Geometry check sheet. Reference: the model listing, model coordinates, mm. Face numbers are marked on the shaded views. A direction names the side the tool comes from. Give positions to 0.01 mm unless a question says otherwise; leave off trailing zeros. Write each loop counter-clockwise with the first axis right and the second up, starting at its lowest first coordinate (ties: lowest second). Pieces come first, ordered by that corner, then holes. Notation, with made-up numbers: M 24.25,60.5 L 83.25,60.5 A22 ccw 83.25,84.5 Z; hole C -16.5,75.5 d2. An arc over 180 degrees is marked long. Write each question's results on one line, items separated by ' | '.
```python
from build123d import *

# Parameters (mm, degrees)
SKETCH_1_R               = 15
SKETCH_1_R_2             = 9
EXTRUDE_1_DEPTH          = 30
SKETCH_2_R               = 100
SKETCH_2_R_2             = 15
SKETCH_2_R_3             = 9
EXTRUDE_2_DEPTH          = 7
CUT_EXTRUDE_1_DEPTH      = 147.181394165
PATTERN_CIRCULAR_1_COUNT = 6
FILLET_1_R               = 10
HOLE_WIZARD_M30_1_D      = 26.5
HOLE_WIZARD_M30_1_DEPTH  = 62.538596798
HOLE_WIZARD_M30_1_TIP    = 7.961403202
CHAMFER_1_SIZE           = 5
CUT_EXTRUDE_1_2_DEPTH    = 145.568322948
PATTERN_CIRCULAR_2_COUNT = 4
FILLET_2_R               = 3


with BuildPart() as part:
    # 草图1 → 凸台-拉伸1 (new body)
    with BuildSketch(Plane(origin=(0, 0, 0), x_dir=(1, 0, 0), z_dir=(0, 1, 0))):
        with Locations(Location((0, 0, 0), (0, 0, 270))):
            Circle(SKETCH_1_R)
        with Locations(Location((0, 0, 0), (0, 0, 270))):
            Circle(SKETCH_1_R_2, mode=Mode.SUBTRACT)
    extrude(amount=EXTRUDE_1_DEPTH)

    # 草图2 → 凸台-拉伸2 (add)
    # profile 1 of 2: a face of its own
    with BuildSketch(Plane(origin=(0, 30, 0), x_dir=(1, 0, 0), z_dir=(0, 1, 0))):
        with Locations(Location((0, 0, 0), (0, 0, 270))):
            Circle(SKETCH_2_R)
        with Locations(Location((0, 0, 0), (0, 0, 270))):
            Circle(SKETCH_2_R_2, mode=Mode.SUBTRACT)
    # profile 2 of 2: a face of its own
    with BuildSketch(Plane(origin=(0, 30, 0), x_dir=(1, 0, 0), z_dir=(0, 1, 0))):
        with Locations(Location((0, 0, 0), (0, 0, 270))):
            Circle(SKETCH_2_R_2)
        with Locations(Location((0, 0, 0), (0, 0, 270))):
            Circle(SKETCH_2_R_3, mode=Mode.SUBTRACT)
    extrude(amount=EXTRUDE_2_DEPTH)

    # 草图7 → Cut-Extrude 1 (cut, through all)
    with BuildSketch(Plane(origin=(0, 37, 0), x_dir=(1, 0, 0), z_dir=(0, 1, 0))):
        with BuildLine():
            Line((-2.5, -10.712142643), (-2.5, 10.712142643))
            ThreePointArc((-2.5, 10.712142643), (0, 11), (2.5, 10.712142643))
            Line((2.5, 10.712142643), (2.5, -10.712142643))
            ThreePointArc((2.5, -10.712142643), (0, -11), (-2.5, -10.712142643))
        make_face()
    cut_extrude_1 = extrude(amount=-CUT_EXTRUDE_1_DEPTH, mode=Mode.SUBTRACT)

    # 阵列(圆周)1: Cut-Extrude 1 ×6 about axis
    pattern_circular_1_axis = Axis((0, 0, 0), (0, 1, 0))
    for i in range(1, PATTERN_CIRCULAR_1_COUNT):
        add(cut_extrude_1.rotate(pattern_circular_1_axis, i * 360 / PATTERN_CIRCULAR_1_COUNT), mode=Mode.SUBTRACT)

    # 圆角1
    fillet_1_edges = [part.edges().sort_by_distance(p)[0] for p in [
        (0, 30, -15),
    ]]
    fillet(fillet_1_edges, radius=FILLET_1_R)

    # M30 螺纹孔1
    with Locations(Plane(origin=(0, 37, 0), x_dir=(1, 0, 0), z_dir=(0, 1, 0))):
        with Locations((0, 62.5), (62.5, 0), (0, -62.5), (-62.5, 0)):
            Hole(HOLE_WIZARD_M30_1_D / 2, depth=HOLE_WIZARD_M30_1_DEPTH)
            with Locations((0, 0, -(HOLE_WIZARD_M30_1_DEPTH + HOLE_WIZARD_M30_1_TIP / 2))):  # 118° drill point
                Cone(0, HOLE_WIZARD_M30_1_D / 2, HOLE_WIZARD_M30_1_TIP, mode=Mode.SUBTRACT)

    # 倒角1
    chamfer_1_edges = [part.edges().sort_by_distance(p)[0] for p in [
        (0, 37, -100),
    ]]
    chamfer(chamfer_1_edges, length=CHAMFER_1_SIZE)

    # 草图10 → Cut-Extrude 1 2 (cut, symmetric)
    with BuildSketch(Plane.XZ.offset(-30)):
        Polygon((30.0520382, -37.830212793), (66.821590822, -74.599765415), (74.599765415, -66.821590822), (37.830212793, -30.0520382), align=None)
    cut_extrude_1_2 = extrude(amount=CUT_EXTRUDE_1_2_DEPTH, both=True, mode=Mode.SUBTRACT)

    # 阵列(圆周)2: Cut-Extrude 1 2 ×4 about axis
    pattern_circular_2_axis = Axis((0, 0, 0), (0, 1, 0))
    for i in range(1, PATTERN_CIRCULAR_2_COUNT):
        add(cut_extrude_1_2.rotate(pattern_circular_2_axis, i * 360 / PATTERN_CIRCULAR_2_COUNT), mode=Mode.SUBTRACT)

    # 圆角2
    fillet_2_edges = [part.edges().sort_by_distance(p)[0] for p in [
        (30.0520382, 33.5, -37.830212793),
        (37.830212793, 33.5, -30.0520382),
        (37.830212793, 33.5, 30.0520382),
        (30.0520382, 33.5, 37.830212793),
        (-30.0520382, 33.5, 37.830212793),
        (-37.830212793, 33.5, 30.0520382),
        (-37.830212793, 33.5, -30.0520382),
        (-30.0520382, 33.5, -37.830212793),
    ]]
    fillet(fillet_2_edges, radius=FILLET_2_R)


solid = part.part
```
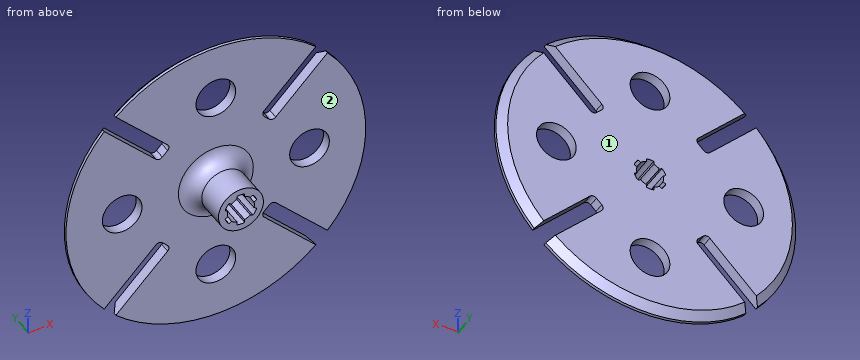
Q1. Section check C-C (z = -56). State how many separate pieces and enclosed holes the cut face has, then the cut area to 3 significant figures.
Answer key:
separate pieces: 4 | enclosed holes: 0 | area: 750 mm2
Q2. Depth check by flat-ended pin: P1, Ø6, axis at x = -64.5, z = -77, coming from the +Y side; P2, Ø6, axis at x = 25, z = -53, coming from the -Y side; P3, Ø1.7, axis at y = 9.5, z = -10, coming from the +X side. Enter the tip coordinate at first touch or a pass-through.
Answer key:
P1: stops at y = 34.55 | P2: stops at y = 30 | P3: stops at x = 11.89
Q3. Access from +Z, -Z, +X, -X, +Y, -Y to the whole of each face (thin tool, end or side, straight path). Record for the marked faces 1 and 2.
Answer key:
face 1: +Z, -Z, +X, -X, +Y | face 2: -Y
Q4. Material ranges on probe 1 along X at (y, z) = (32, -62.5); probe 2 along X at (y, z) = (32, -62); probe 3 along X at (y, z) = (13, 1), recorded low to high. Write a range as [from, to].
Answer key:
probe 1: x = [-78.06, -70.28], [-54.72, -13.25], [13.25, 54.72], [70.28, 78.06] | probe 2: x = [-78.46, -69.78], [-54.22, -13.24], [13.24, 54.22], [69.78, 78.46] | probe 3: x = [-14.97, -8.94], [8.94, 14.97]
Q5. Section check A-A (y = 17). Enter the section's corners in (x, z), then the cut area to 3 significant figures.
Answer key:
outline: C 0,0 d30; hole M -10.53,-3.19 A11 ccw -8.03,-7.52 L -6.24,-6.49 A9 ccw -2.5,-8.65 L -2.5,-10.71 A11 ccw 2.5,-10.71 L 2.5,-8.65 A9 ccw 6.24,-6.49 L 8.03,-7.52 A11 ccw 10.53,-3.19 L 8.74,-2.16 A9 ccw 8.74,2.16 L 10.53,3.19 A11 ccw 8.03,7.52 L 6.24,6.49 A9 ccw 2.5,8.65 L 2.5,10.71 A11 ccw -2.5,10.71 L -2.5,8.65 A9 ccw -6.24,6.49 L -8.03,7.52 A11 ccw -10.53,3.19 L -8.74,2.16 A9 ccw -8.74,-2.16 Z | area: 392 mm2
Q6. Section check B-B (x = 0). Enter the section's corners in (y, z), then the cut area to 3 significant figures.
Answer key:
outline: M 0,-15 L 20,-15 A10 cw 30,-25 L 30,-49.25 L 37,-49.25 L 37,-11 L 0,-11 Z; M 0,11 L 37,11 L 37,49.25 L 30,49.25 L 30,25 A10 cw 20,15 L 0,15 Z; M 30,-100 L 32,-100 L 37,-95 L 37,-75.75 L 30,-75.75 Z; M 30,75.75 L 37,75.75 L 37,95 L 32,100 L 30,100 Z | area: 1,130 mm2
